Drawing for the job (mm, zero at the part's lowest x, y, z). Give positions to 0.01 mm unless a question says otherwise; leave off trailing zeros. Order: outer loops, then holes, each group sorted by start corner. A loop starts at its lowest first (then second) coordinate and runs counter-clockwise, first axis right, second up. Notation, with made-up numbers: (57, 27.25) - (66, 27.25) arc R22 ccw to (66, 54.25) - close; hole circle Ø7 at (-35, 40.5). An arc over 180 degrees is marked (long way). Use a Markdown table: item, result.
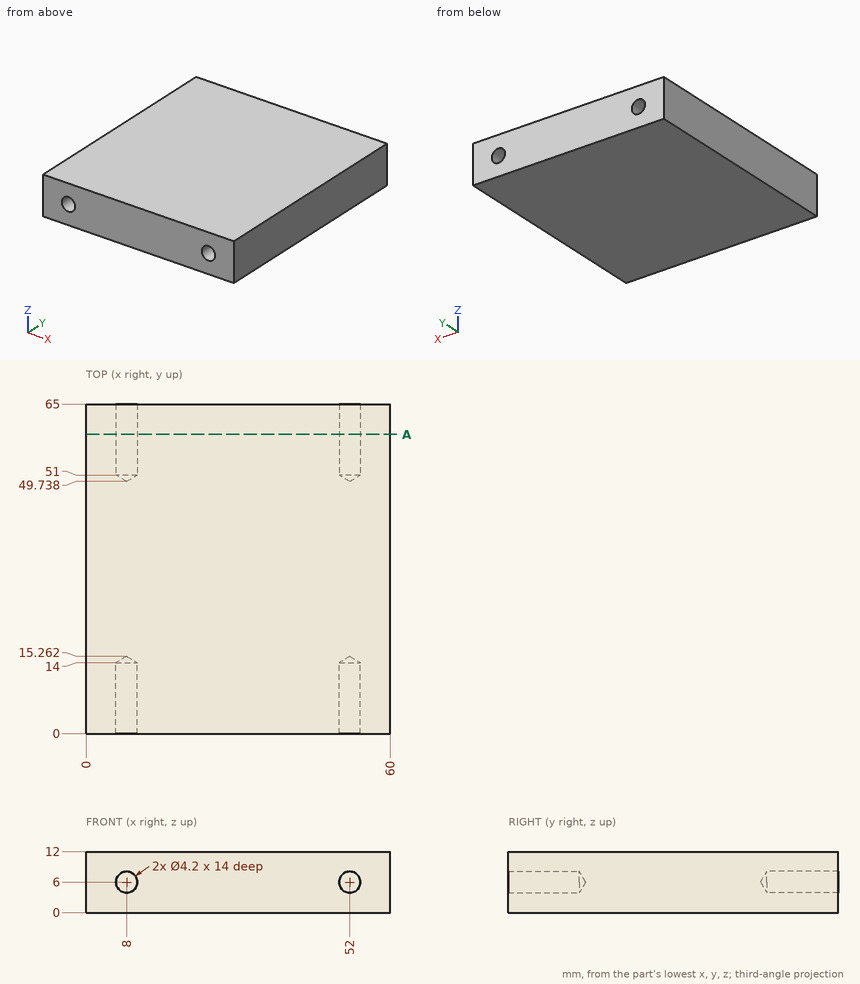
1) Pin check, flat tips, straight feed: P1, Ø4, axis at x = 8, z = 6, coming from the -Y side; P2, Ø4, axis at x = 52, z = 6, coming from the +Y side. Stop position of each tip, or through.
Computed:
| item | result |
|---|---|
| P1 | stops at y = 14.06 |
| P2 | stops at y = 50.94 |
2) Slice it at A-A (y = 59). Write the cut outline in (x, z).
Computed:
| item | result |
|---|---|
| outline | (0, 0) - (60, 0) - (60, 12) - (0, 12) - close; hole circle Ø4.2 at (8, 6); hole circle Ø4.2 at (52, 6) |
3) Wall check: line 1 (X direction, y = 10, z = 6); line 2 (Z direction, x = 8, y = 9). Give the ranges that are in metal, low to high. Write a range as from..to.
Computed:
| item | result |
|---|---|
| line 1 | x = 0..5.9, 10.1..49.9, 54.1..60 |
| line 2 | z = 0..3.9, 8.1..12 |
